from build123d import *

# Parameters (mm, degrees)
SKETCH_1_R         = 1.5
EXTRUDE_1_DEPTH    = 8.5
SKETCH_1_3_R       = 1.5
EXTRUDE_2_DEPTH    = 3
EXTRUDE_START      = 11.5
SKETCH_1_4_R       = 1.5
EXTRUDE_3_DEPTH    = 11.5
HOLE_WIZARD_M6_1_D = 5
FILLET_1_R         = 0.3


with BuildPart() as part:
    # 스케치1 → 보스-돌출1 (new body)
    # profile 1 of 3: a face of its own
    with BuildSketch(Plane.XY):
        Polygon((8.939511347, -1.33586653), (8.939511347, -8.29586653), (-6.060488653, -8.29586653), (-6.060488653, 5.62413347), (1.439511347, 5.62413347), align=None)
        with Locations((3.939511347, -1.33586653)):
            Circle(SKETCH_1_R, mode=Mode.SUBTRACT)
        with Locations((-2.060488653, -1.33586653)):
            Circle(SKETCH_1_R, mode=Mode.SUBTRACT)
    # profile 2 of 3: a face of its own
    with BuildSketch(Plane.XY):
        with Locations((3.939511347, -1.33586653)):
            Circle(SKETCH_1_R)
    # profile 3 of 3: a face of its own
    with BuildSketch(Plane.XY):
        with Locations((-2.060488653, -1.33586653)):
            Circle(SKETCH_1_R)
    extrude(amount=EXTRUDE_1_DEPTH)

    # 스케치1<3> → 보스-돌출2 (add)
    with BuildSketch(Plane.XY):
        with Locations((3.939511347, -1.33586653)):
            Circle(SKETCH_1_3_R)
        with Locations((-2.060488653, -1.33586653)):
            Circle(SKETCH_1_3_R)
    extrude(amount=-EXTRUDE_2_DEPTH)

    # 스케치1<4> → 보스-돌출3 (add)
    with BuildSketch(Plane.XY.offset(EXTRUDE_START)):
        with Locations((-2.060488653, -1.33586653)):
            Circle(SKETCH_1_4_R)
        with Locations((3.939511347, -1.33586653)):
            Circle(SKETCH_1_4_R)
    extrude(amount=-EXTRUDE_3_DEPTH)

    # M6 탭을 위한 탭 드릴1 (through all)
    with Locations(Plane(origin=(1.439511347, -8.29586653, 4.25), x_dir=(0, 0, -1), z_dir=(0, -1, 0))):
        with Locations((0, 0)):
            Hole(HOLE_WIZARD_M6_1_D / 2)

    # 필렛1
    fillet_1_edges = [part.edges().sort_by_distance(p)[0] for p in [
        (2.439511347, -1.33586653, -3),
        (-3.560488653, -1.33586653, -3),
        (-3.560488653, -1.33586653, 11.5),
        (2.439511347, -1.33586653, 11.5),
    ]]
    fillet(fillet_1_edges, radius=FILLET_1_R)


solid = part.part
The listing builds one solid part. Answer for the finished solid, in the listing's coordinates (mm). A direction names the side the tool comes from. Coordinates: 2 decimals unless noted, no trailing zeros. Order: outer loops, then holes, each group sorted by start corner. A loop starts at its lowest first (then second) coordinate and runs counter-clockwise, first axis right, second up. Notation, with made-up numbers: (26.25, -37.75) -> (81.25, -37.75) arc R21 cw to (81.25, -7.75) -> close; hole circle Ø6 at (15, 83). An arc over 180 degrees is marked (long way). Answer in a Markdown table with one row per item. Add a question column.
Item 1: Find section D-D (y = 3). Write down the section's boundary in (x, z), then the cut area to 3 significant figures.
Item 2: Find section B-B (x = 0). Write down the section's boundary in (y, z), then the cut area to 3 significant figures.
Item 3: Find the intervals of material crossed by L1, parallel to X at y = -5.5, z = 4.25; L2, parallel to Z at x = -5, y = 0.25; L3, parallel to Z at x = -0.5, y = 5.25, in increasing order. Write a range as from..to.
Item 4: This flat-tipped pin is pushed along its axis until it touches: P1, Ø5, axis at x = 2.5, y = -5.5, coming from the -Z side. Where does it stop, or does it pass through?
Item 5: Find section C-C (z = 3). Write down the section's boundary in (x, y).
Item 6: Determine the mould class of faces 1 (the face through (-3.25, -2.25, -1.33)), 2 (the face through (-2, -1, 11.5)), 3 (the face through (-1, -1.2, 3.7)) for opening direction Z: +Z half, -Z half, draft (parallel to the pull), parting line (faces both ways), or undercut.
Item 7: Find section A-A (y = -5.25). Write down the section's boundary in (x, z), then the cut area to 3 significant figures.
Item 8: Which of the six approach directions +Z, -Z, +X, -X, +Y, -Y give full straight-line access (tool end or side, diameter ignored) to faces 4 (the face through (3, -8.296, 2)), 5 (the face through (3.61, -2.8, 9.87)), 6 (the face through (3.61, -2.8, -1.33))?
Result set:
| question | item | result |
|---|---|---|
| 1 | outline | (-6.06, 0) -> (4.27, 0) -> (4.27, 8.5) -> (-6.06, 8.5) -> close; hole circle Ø5 at (1.44, 4.25) |
| 1 | area | 68.2 mm² |
| 2 | outline | (-8.3, 0) -> (5.62, 0) -> (5.62, 2.21) -> (-8.3, 2.21) -> close; (-8.3, 6.29) -> (5.62, 6.29) -> (5.62, 8.5) -> (-8.3, 8.5) -> close |
| 2 | area | 61.4 mm² |
| 3 | L1 | x = -6.06..-1.06, 3.94..8.94 |
| 3 | L2 | z = 0..8.5 |
| 3 | L3 | z = 0..2.67, 5.83..8.5 |
| 4 | P1 | stops at z = 0 |
| 5 | outline | (-6.06, -8.3) -> (-0.73, -8.3) -> (-0.73, 5.62) -> (-6.06, 5.62) -> close; (3.6, -8.3) -> (8.94, -8.3) -> (8.94, -1.34) -> (3.6, 3.61) -> close |
| 6 | face 1 | draft |
| 6 | face 2 | +Z half |
| 6 | face 3 | undercut |
| 7 | outline | (-6.06, 0) -> (8.94, 0) -> (8.94, 8.5) -> (-6.06, 8.5) -> close; hole circle Ø5 at (1.44, 4.25) |
| 7 | area | 108 mm² |
| 8 | face 4 | +Z, -Z, +X, -X, -Y |
| 8 | face 5 | +Z |
| 8 | face 6 | -Z |
